Geometry check sheet. Reference: the model listing, model coordinates, mm. A direction names the side the tool comes from. Round coordinates to 2 decimals unless told otherwise and drop trailing zeros. Loops run counter-clockwise (first coordinate to the right, second up) from the corner with the lowest first, then second, coordinate; pieces in that order, holes last. Notation, with made-up numbers: (-18.75, 85) - (4.25, 85) arc R32 cw to (4.25, 118) - close; hole circle Ø3 at (28.25, -38). An arc over 180 degrees is marked (long way). Answer as CSV lines item,"result". Start each with the question number.
1) Cross-section at B-B on x = -26. Record the boundary of the cut face in (y, z).
2) Access from +Z, -Z, +X, -X, +Y, -Y to the whole of each face (thin tool, end or side, straight path). Record for faces 5 (the flat face through (-5.525, 3.131, 12.522)), 6 (the flat face through (8, 1, 25.4)).
3) Cross-section at A-A on z = 2.75. Record the boundary of the cut face in (x, y), and give its area (3 significant figures).
4) Thickness scan on line 1 along X through (y, z) = (2, 3); line 2 along X through (y, z) = (-4.5, 18.25); line 3 along X through (y, z) = (-33, 4.25). Record the ranges inside material, lowest first.
5) Draft check along Y on faces 1 (the flat face through (8, 1, 0)), 2 (the cylindrical face through (-30.235, 23.183, 12.522)), 3 (the flat face through (5.474, 3.219, 12.522)), 4 (the flat face through (0, 6.35, 13)). Enter one of: released by +Y, released by -Y, zero draft, split by the parting line, or undercut.
6) Cross-section at C-C on y = -16. Record the boundary of the cut face in (x, z), and give its area (3 significant figures).
7) Depth check by flat-ended pin: P1, Ø1.5, axis at y = 20, z = 10.5, coming from the +X side; P2, Ø2, axis at x = -30.5, z = 16, coming from the -Y side; P3, Ø5, axis at x = -4, z = 8, coming from the +Y side. Enter the tip coordinate at first touch or a pass-through.
Autodesk Inventor part; units mm, degrees
ref_plane "YZ Plane" through (0, 0, 0) normal (1, 0, 0) x (0, 1, 0)
ref_plane "XZ Plane" through (0, 0, 0) normal (0, 1, 0) x (-1, 0, 0)
ref_plane "XY Plane" through (0, 0, 0) normal (0, 0, 1) x (1, 0, 0)
sketch "Sketch1" plane through (0, 0, 0) normal (0, 0, 1) x (1, 0, 0)
  circle A0 centre (0, 0) radius 38.1
  line L0 (3.6662, 6.35) -> (7.3323, 0)
  line L1 (7.3323, 0) -> (3.6662, -6.35)
  line L2 (3.6662, -6.35) -> (-3.6662, -6.35)
  line L3 (-3.6662, -6.35) -> (-7.3323, 0)
  line L4 (-7.3323, 0) -> (-3.6662, 6.35)
  line L5 (-3.6662, 6.35) -> (3.6662, 6.35)
  line L6 (0, 0) -> (-13.8069, 0)
  dimension "d0" = 76.2
  dimension "d1" = 12.7
extrude "Extrusion1" add sketch "Sketch1" along normal blind 25.4
properties part number "Simple 3 in wheel"
Answer block:
1,outline,"(-27.85, 0) - (27.85, 0) - (27.85, 25.4) - (-27.85, 25.4) - close"
2,face 5,"+Z, -Z"
2,face 6,"+Z, +X, -X, +Y, -Y"
3,outline,"circle Ø76.2 at (0, 0); hole (-7.33, 0) - (-3.67, -6.35) - (3.67, -6.35) - (7.33, 0) - (3.67, 6.35) - (-3.67, 6.35) - close"
3,area,"4,420 mm^2"
4,line 1,"x = -38.05 to -6.18, 6.18 to 38.05"
4,line 2,"x = -37.83 to -4.73, 4.73 to 37.83"
4,line 3,"x = -19.04 to 19.04"
5,face 1,"zero draft"
5,face 2,"split by the parting line"
5,face 3,"undercut"
5,face 4,"undercut"
6,outline,"(-34.58, 0) - (34.58, 0) - (34.58, 25.4) - (-34.58, 25.4) - close"
6,area,"1,760 mm^2"
7,P1,"stops at x = 32.88"
7,P2,"stops at y = -24.11"
7,P3,"stops at y = 38.07"
